Input: dimensioned drawing with shaded views. Units: mm. Origin: part minimum x, y, z. Round coordinates to 2 decimals unless told otherwise and drop trailing zeros. Loops run counter-clockwise (first coordinate to the right, second up) from the corner with the lowest first, then second, coordinate; pieces in that order, holes last. Notation, with made-up numbers: (-24.75, 5.5) - (30.25, 5.5) arc R12 cw to (30.25, 17.5) - close; hole circle Ø9 at (37.5, 22.5). An arc over 180 degrees is marked (long way). One line per question, with ' | ' between items. Start each with the question number.
1. Pin query (flat end, axial travel): pin 1 (1.3 mm diameter, centred on y = 1.5, z = 56.5, fed in from +X). Return the tip coordinate at first contact, or that it passes through.
2. Ray query, line 1 (X direction, y = 0.5, z = 104) (1 decimal); line 2 (X direction, y = 1.5, z = 105); line 3 (Z direction, x = 24, y = 0.7). Return the intervals inside material, ascending.
3. Cut plane B-B (y = 1.75). Return loops of the section in (x, z), then the cut area to 3 significant figures.
4. Cut plane C-C (x = 15). Return loops of the section in (y, z).
5. Cut plane A-A (z = 65.5). Return loops of the section in (x, y), then the cut area to 3 significant figures.
6. Cut plane D-D (z = 24.5). Return loops of the section in (x, y).
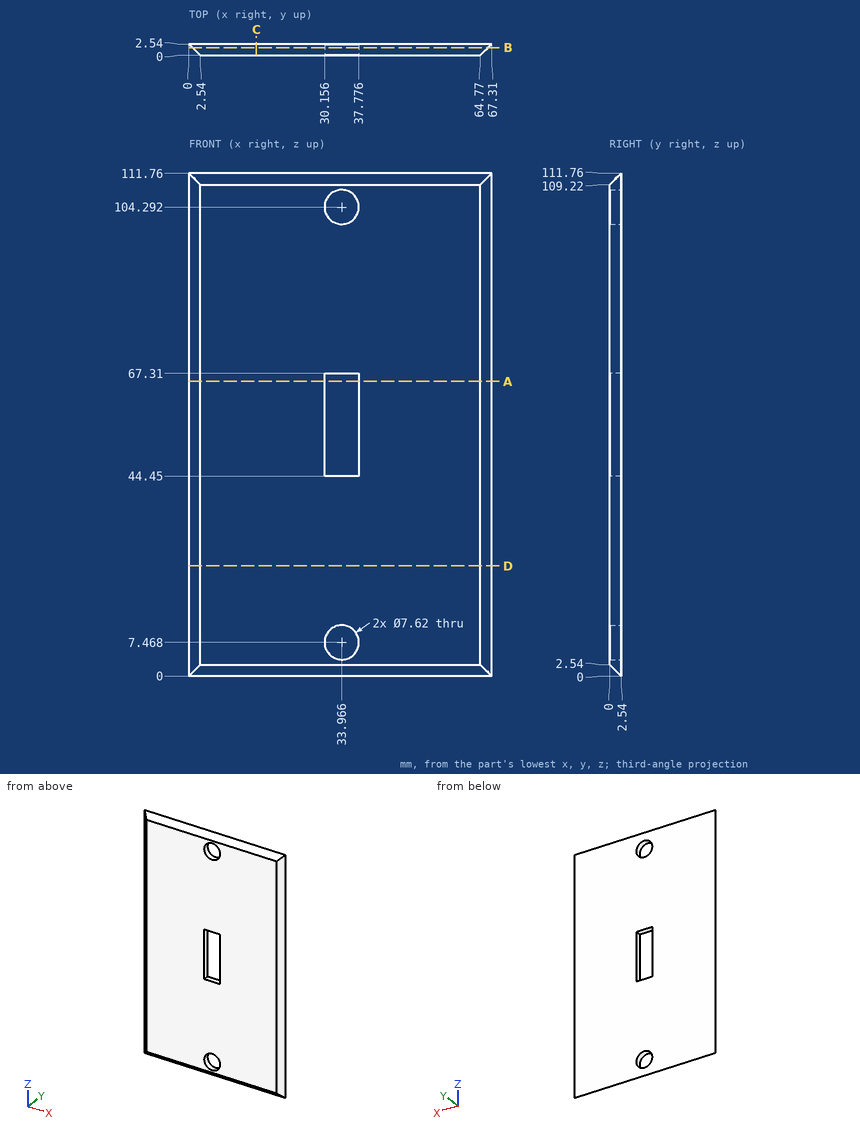
Answers follow:
1) pin 1: stops at x = 66.92
2) line 1: x = 2 to 30.2, 37.8 to 65.3 | line 2: x = 1.04 to 30.22, 37.71 to 66.27 | line 3: z = 1.84 to 109.92
3) outline: (0.79, 0.79) - (66.52, 0.79) - (66.52, 110.97) - (0.79, 110.97) - close; hole circle Ø7.62 at (33.97, 7.47); hole (30.16, 44.45) - (37.78, 44.45) - (37.78, 67.31) - (30.16, 67.31) - close; hole circle Ø7.62 at (33.97, 104.29) | area: 6,980 mm2
4) outline: (0, 2.54) - (2.54, 0) - (2.54, 111.76) - (0, 109.22) - close
5) outline: (0, 2.54) - (2.54, 0) - (30.16, 0) - (30.16, 2.54) - close; (37.78, 0) - (64.77, 0) - (67.31, 2.54) - (37.78, 2.54) - close | area: 145 mm2
6) outline: (0, 2.54) - (2.54, 0) - (64.77, 0) - (67.31, 2.54) - close
